Input: part model. Units: mm. Frame: model coordinates. Coordinates: 2 decimals unless noted, no trailing zeros. Write each loop counter-clockwise with the first axis right and the second up, starting at its lowest first coordinate (ties: lowest second). Pieces come first, ordered by that corner, then holes. Notation, with made-up numbers: (40.25, -22) - (80.25, -22) arc R36 ccw to (80.25, 14) - close; hole circle Ø2 at (-6.5, 59). An arc over 180 degrees is marked (long way). One line per question, with ' | ' between items. Start each with the question number.
1) First-contact query: P1, Ø8, axis at x = 4.5, z = 43, coming from the +Y side; P2, Ø16, axis at x = -4.5, y = -828.5, coming from the +Z side; P3, Ø5, axis at y = -1925.5, z = 36, coming from the +X side; P4, Ø16, axis at x = 6.5, y = -2171, coming from the +Z side. Flat tips, straight axial feed; report the tip coordinate or a pass-through.
2) Line query: line 1 (Y direction, x = 6, z = 19); line 2 (Z direction, x = 3, y = -257). Output: solid intervals per line, ascending.
3) Section query A-A on y = -822. Return loops of the section in (x, z), and give its area (3 significant figures).
```python
from build123d import *

# Parameters (mm, degrees)
F0_W     = 32
F0_H     = 32
F1_DEPTH = 2208
F3_W     = 32
F3_H     = 32
F4_DEPTH = 2100
F5_W     = 55
F5_H     = 20
F6_DEPTH = 32


with BuildPart() as f1:
    # F0 (on Front) → F1 (new body)
    with BuildSketch(Plane.XZ):
        Rectangle(F0_W, F0_H)
    extrude(amount=F1_DEPTH)

    # F3 (on offset) → F4 (join)
    with BuildSketch(Plane.XZ.offset(50)):
        with Locations((0, 32)):
            Rectangle(F3_W, F3_H)
    extrude(amount=F4_DEPTH)

    # F5 (on face) → F6 (cut)
    with BuildSketch(Plane.YZ.offset(16)):
        with Locations((-107.5, 42)):
            Rectangle(F5_W, F5_H)
        with Locations((-187.5, 42)):
            Rectangle(F5_W, F5_H)
        with Locations((-267.5, 42)):
            Rectangle(F5_W, F5_H)
        with Locations((-347.5, 42)):
            Rectangle(F5_W, F5_H)
        with Locations((-427.5, 42)):
            Rectangle(F5_W, F5_H)
        with Locations((-507.5, 42)):
            Rectangle(F5_W, F5_H)
        with Locations((-587.5, 42)):
            Rectangle(F5_W, F5_H)
        with Locations((-667.5, 42)):
            Rectangle(F5_W, F5_H)
        with Locations((-747.5, 42)):
            Rectangle(F5_W, F5_H)
        with Locations((-827.5, 42)):
            Rectangle(F5_W, F5_H)
        with Locations((-907.5, 42)):
            Rectangle(F5_W, F5_H)
        with Locations((-987.5, 42)):
            Rectangle(F5_W, F5_H)
        with Locations((-1067.5, 42)):
            Rectangle(F5_W, F5_H)
        with Locations((-1147.5, 42)):
            Rectangle(F5_W, F5_H)
        with Locations((-1227.5, 42)):
            Rectangle(F5_W, F5_H)
        with Locations((-1307.5, 42)):
            Rectangle(F5_W, F5_H)
        with Locations((-1387.5, 42)):
            Rectangle(F5_W, F5_H)
        with Locations((-1467.5, 42)):
            Rectangle(F5_W, F5_H)
        with Locations((-1547.5, 42)):
            Rectangle(F5_W, F5_H)
        with Locations((-1627.5, 42)):
            Rectangle(F5_W, F5_H)
        with Locations((-1707.5, 42)):
            Rectangle(F5_W, F5_H)
        with Locations((-1787.5, 42)):
            Rectangle(F5_W, F5_H)
        with Locations((-1867.5, 42)):
            Rectangle(F5_W, F5_H)
        with Locations((-1947.5, 42)):
            Rectangle(F5_W, F5_H)
        with Locations((-2027.5, 42)):
            Rectangle(F5_W, F5_H)
    extrude(amount=-F6_DEPTH, mode=Mode.SUBTRACT)


solid = f1.part
```
Answer key:
1) P1: y = -50 | P2: z = 32 | P3: through | P4: z = 16
2) line 1: -2150 to -50 | line 2: -16 to 32
3) outline: (-16, -16) - (16, -16) - (16, 32) - (-16, 32) - close | area: 1,540 mm²
